Work out the finished part from the listing and answer in its coordinate system (mm). Face numbers are marked on the shaded views. A direction names the side the tool comes from. Give positions to 0.01 mm unless a question says otherwise; leave off trailing zeros. Loops run counter-clockwise (first coordinate to the right, second up) from the corner with the lowest first, then second, coordinate; pieces in that order, holes last. Notation, with made-up numbers: M -30.5,-9.5 L -8.5,-9.5 A23 cw -8.5,9.5 Z; hole C 70,63 d5. An arc over 180 degrees is marked long. Use a Markdown table: item, result.
```python
from build123d import *

# Parameters (mm, degrees)
SKETCH1_R                         = 20.6375
BOSS_EXTRUDE1_DEPTH               = 4.7625
SKETCH2_R                         = 8.73125
BOSS_EXTRUDE2_DEPTH               = 6.096
SKETCH5_R                         = 4.7625
BOSS_EXTRUDE3_DEPTH               = 28.575
F_1_4_20_TAPPED_HOLE2_D           = 5.1054
F_1_4_20_TAPPED_HOLE2_DEPTH       = 29.21
F_1_4_20_TAPPED_HOLE2_CBORE_D     = 6.35
F_1_4_20_TAPPED_HOLE2_CBORE_DEPTH = 25.4
F_1_4_20_TAPPED_HOLE2_TIP         = 1.533816902
F_10_32_TAPPED_HOLE1_D            = 4.0386
SKETCH11_R                        = 6.35
BOSS_EXTRUDE4_DEPTH               = 9.525
FILLET1_R                         = 3.175


with BuildPart() as part:
    # Sketch1 → Boss-Extrude1 (new body)
    with BuildSketch(Plane(origin=(0, 0, 0), x_dir=(1, 0, 0), z_dir=(0, 1, 0))):
        Circle(SKETCH1_R)
    extrude(amount=BOSS_EXTRUDE1_DEPTH)

    # Sketch2 → Boss-Extrude2 (add)
    with BuildSketch(Plane.XZ):
        Circle(SKETCH2_R)
    extrude(amount=BOSS_EXTRUDE2_DEPTH)

    # Sketch5 → Boss-Extrude3 (add)
    with BuildSketch(Plane.XZ.offset(6.096)):
        Circle(SKETCH5_R)
    extrude(amount=BOSS_EXTRUDE3_DEPTH)

    # 1/4-20 Tapped Hole2
    with Locations(Plane(origin=(0, -34.671, 0), x_dir=(-1, 0, 0), z_dir=(0, -1, 0))):
        with Locations((0, 0)):
            CounterBoreHole(F_1_4_20_TAPPED_HOLE2_D / 2, F_1_4_20_TAPPED_HOLE2_CBORE_D / 2, F_1_4_20_TAPPED_HOLE2_CBORE_DEPTH, depth=F_1_4_20_TAPPED_HOLE2_DEPTH)
            with Locations((0, 0, -(F_1_4_20_TAPPED_HOLE2_DEPTH + F_1_4_20_TAPPED_HOLE2_TIP / 2))):  # 118° drill point
                Cone(0, F_1_4_20_TAPPED_HOLE2_D / 2, F_1_4_20_TAPPED_HOLE2_TIP, mode=Mode.SUBTRACT)

    # #10-32 Tapped Hole1 (through all)
    with Locations(Plane(origin=(0, 0, 0), x_dir=(-1, 0, 0), z_dir=(0, -1, 0))):
        with Locations((-13.748153285, -7.9375), (0, 15.875), (13.748153285, -7.9375)):
            Hole(F_10_32_TAPPED_HOLE1_D / 2)

    # Sketch11 → Boss-Extrude4 (add)
    with BuildSketch(Plane(origin=(0, 4.7625, 0), x_dir=(1, 0, 0), z_dir=(0, 1, 0))):
        Circle(SKETCH11_R)
    extrude(amount=BOSS_EXTRUDE4_DEPTH)

    # Fillet1
    fillet1_edges = [part.edges().sort_by_distance(p)[0] for p in [
        (-6.35, 4.7625, 0),
    ]]
    fillet(fillet1_edges, radius=FILLET1_R)


solid = part.part
```
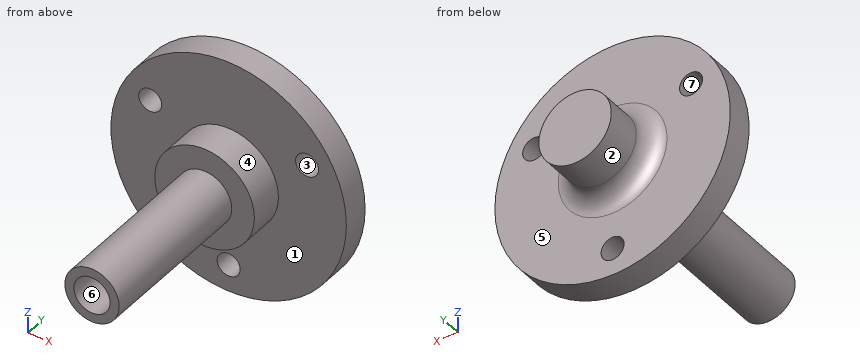
(1) Which of the six approach directions +Z, -Z, +X, -X, +Y, -Y give full straight-line access (tool end or side, diameter ignored) to the marked faces 1, 2 and 3?
Entries:
| item | result |
|---|---|
| face 1 | -Y |
| face 2 | +Y |
| face 3 | +Y, -Y |
(2) Consider probe 1 along Z at (x, y) = (0, -6); probe 2 along Z at (x, y) = (0, -28) (1 decimal); probe 3 along Y at (x, z) = (-6, 0.5). Determine where each line is inside the solid, lowest interval first. Write a range as [from, to].
Entries:
| item | result |
|---|---|
| probe 1 | z = [-8.73, -2.55], [2.55, 8.73] |
| probe 2 | z = [-4.8, -3.2], [3.2, 4.8] |
| probe 3 | y = [-6.1, 14.29] |
(3) A cutting plane is placed at C-C (z = 16). Write down the section's boundary in (x, y).
Entries:
| item | result |
|---|---|
| outline | M -13.03,0 L 13.03,0 L 13.03,4.76 L -13.03,4.76 Z |
(4) Given P1, Ø1.5, axis at y = -18.5, z = 2, coming from the -X side; P2, Ø3.5, axis at x = 0, z = -15.875, coming from the -Y side; P3, Ø12, axis at y = -23.5, z = -0.5, coming from the +X side; P4, Ø7.5, axis at x = 0, z = 0, coming from the -Y side, each flat-ended and moving along its own axis, determine where each tip first touches the part or whether it passes through.
Entries:
| item | result |
|---|---|
| P1 | stops at x = -4.6 |
| P2 | passes through |
| P3 | stops at x = 4.76 |
| P4 | stops at y = -34.67 |
(5) A cutting plane is placed at B-B (y = -1). Write down the section's boundary in (x, z).
Entries:
| item | result |
|---|---|
| outline | C 0,0 d17.46 |
(6) The mould has two halves that part along X. Classify the marked faces 4, 5, 6 and 7: released by +X, released by -X, zero draft, split by the parting line, or undercut.
Entries:
| item | result |
|---|---|
| face 4 | split by the parting line |
| face 5 | zero draft |
| face 6 | undercut |
| face 7 | undercut |
